from build123d import *

# Parameters (mm, degrees)
SKETCH2_W           = 30
SKETCH2_H           = 30
SKETCH2_R           = 1.2192
BOSS_EXTRUDE1_DEPTH = 1.5875
CUT_EXTRUDE1_DEPTH  = 22.272521154


with BuildPart() as part:
    # Sketch2 → Boss-Extrude1 (new body)
    with BuildSketch(Plane.XY):
        Rectangle(SKETCH2_W, SKETCH2_H)
        with Locations((-10, 12.38905)):
            Circle(SKETCH2_R, mode=Mode.SUBTRACT)
        with Locations((10, 12.38905)):
            Circle(SKETCH2_R, mode=Mode.SUBTRACT)
        with Locations((10, -12.38905)):
            Circle(SKETCH2_R, mode=Mode.SUBTRACT)
        with Locations((-10, -12.38905)):
            Circle(SKETCH2_R, mode=Mode.SUBTRACT)
    extrude(amount=BOSS_EXTRUDE1_DEPTH)

    # Sketch3 → Cut-Extrude1 (cut, through all)
    with BuildSketch(Plane(origin=(0, 0, 0), x_dir=(-1, 0, 0), z_dir=(0, 0, -1))):
        with BuildLine():
            Line((-11.825, -1.5875), (-15, -1.5875))
            Line((-15, -1.5875), (-15, 1.5875))
            Line((-15, 1.5875), (-11.825, 1.5875))
            ThreePointArc((-11.825, 1.5875), (-10.2375, 0), (-11.825, -1.5875))
        make_face()
    extrude(amount=-CUT_EXTRUDE1_DEPTH, mode=Mode.SUBTRACT)


solid = part.part
Model file for the job. Use its own axes, mm. A direction names the side the tool comes from. Coordinates: 2 decimals unless noted, no trailing zeros. Loops run counter-clockwise (first coordinate to the right, second up) from the corner with the lowest first, then second, coordinate; pieces in that order, holes last. Notation, with made-up numbers: (-27, -18) -> (32, -18) arc R36 ccw to (32, 20) -> close; hole circle Ø3 at (-40, 70.25). An arc over 180 degrees is marked (long way). Use one line per item in the form item = value. Start each with the question number.
(1) Flat gauge pin, fed straight in: pin 1 (2 mm diameter, centred on x = 10, y = 12.39, fed in from +Z). Where does the tip first touch, or does it go through?
(2) Cut at A-A on x = -10. Give the cut face in (y, z).
(3) Probe probe 1 along Y at (x, z) = (10, 1.25); probe 2 along X at (y, z) = (-12.5, 0.65); probe 3 along Y at (x, z) = (12.25, 0.45). List the from-to ranges inside material, lowest first. Write a range as from..to.
(4) Cut at C-C on y = 0. Give the cut face in (x, z), and give its area (3 significant figures).
(5) Cut at B-B on z = 1.2. Give the cut face in (x, y) (1 decimal).
(6) Pull direction X, two halves, no side cores. Call faces 3 (the flat face through (-15, 0, 1)), 4 (the flat face through (0, 15, 1)), 5 (the cylindrical face through (-10.264, 11.199, 0.783)), 6 (the cylindrical face through (9.03, 11.65, 0.78)): pulls with the +X half, pulls with the -X half, needs draft (parallel to the pull), parting line crosses it, or undercut.
(7) Tool access for faces 1 (the flat face through (13, -1.588, 1)), 2 (the cylindrical face through (-10.97, -13.13, 0.78)): list every direction of +Z, -Z, +X, -X, +Y, -Y with a clear straight run to the whole face (end or side of a thin tool).
Values:
q1.pin_1 = through
q2.outline = (-15, 0) -> (-13.61, 0) -> (-13.61, 1.59) -> (-15, 1.59) -> close; (-11.17, 0) -> (11.17, 0) -> (11.17, 1.59) -> (-11.17, 1.59) -> close; (13.61, 0) -> (15, 0) -> (15, 1.59) -> (13.61, 1.59) -> close
q3.probe_1 = -15..-13.61, -11.17..11.17, 13.61..15
q3.probe_2 = -15..-11.21, -8.79..8.79, 11.21..15
q3.probe_3 = -15..-1.59, 1.59..15
q4.outline = (-15, 0) -> (10.24, 0) -> (10.24, 1.59) -> (-15, 1.59) -> close
q4.area = 40.1 mm2
q5.outline = (-15, -15) -> (15, -15) -> (15, -1.6) -> (11.8, -1.6) arc R1.6 cw to (11.8, 1.6) -> (15, 1.6) -> (15, 15) -> (-15, 15) -> close; hole circle Ø2.4 at (-10, -12.4); hole circle Ø2.4 at (-10, 12.4); hole circle Ø2.4 at (10, -12.4); hole circle Ø2.4 at (10, 12.4)
q6.face_3 = pulls with the -X half
q6.face_4 = needs draft
q6.face_5 = undercut
q6.face_6 = undercut
q7.face_1 = +Z, -Z, +X
q7.face_2 = +Z, -Z
